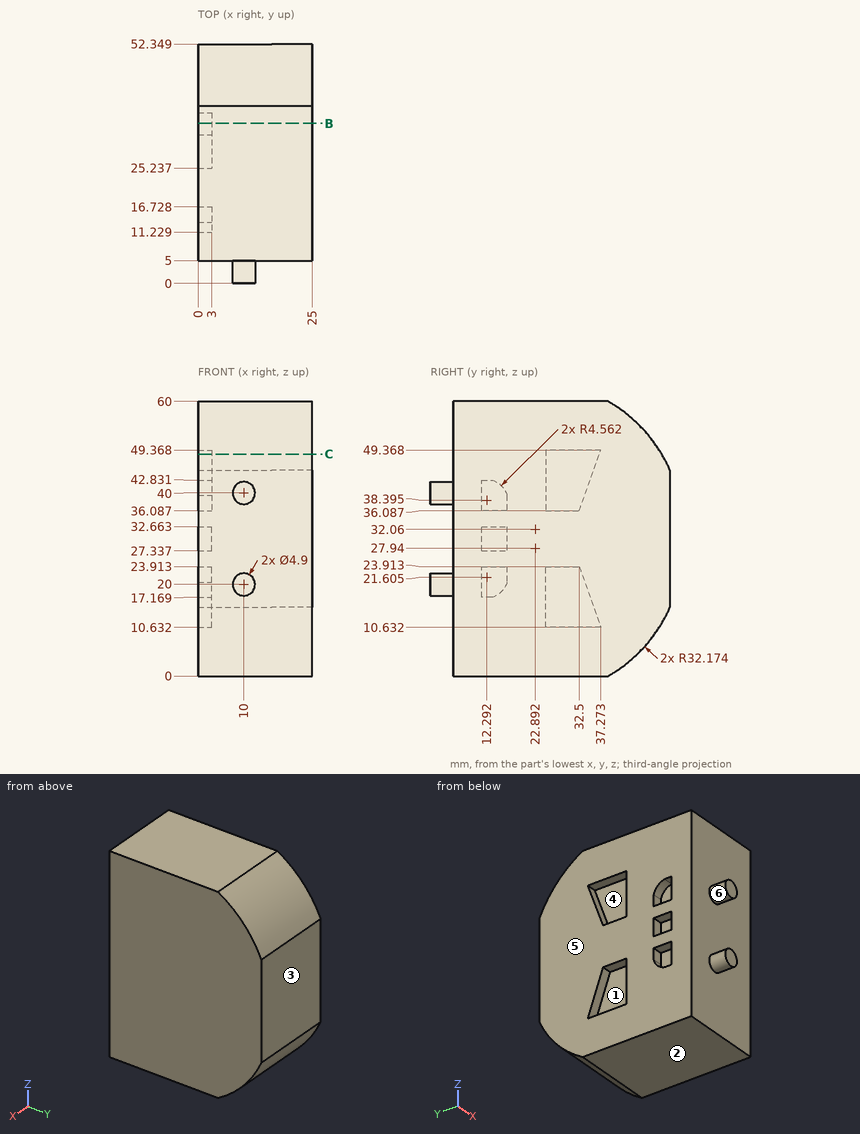
Study the drawing (mm; zero at the part's minimum x, y, z) and answer. A direction names the side the tool comes from. Give positions to 0.01 mm unless a question says otherwise; leave off trailing zeros. Loops run counter-clockwise (first coordinate to the right, second up) from the corner with the lowest first, then second, coordinate; pieces in that order, holes last. Notation, with made-up numbers: (-21, 84.25) - (-8, 84.25) arc R15 ccw to (-8, 109.25) - close; hole circle Ø4 at (55, 18). An arc over 180 degrees is marked (long way). Return JSON: item names as keys, results as strings. Group by question number.
1. Given pin 1 Ø1.5 at (x, z) = (13.5, 30.5) entering from -Y; pin 2 Ø3.5 at (y, z) = (31.5, 41) entering from -X; pin 3 Ø2 at (x, z) = (14, 46.5) entering from +Y (1 decimal), each flat-ended and moving along its own axis, determine where each tip first touches the part or whether it passes through.
2. Straight lines are drawn through the part: line 1 (Y direction, x = 2.25, z = 37.5); line 2 (Y direction, x = 2, z = 11) (1 decimal); line 3 (Y direction, x = 21.5, z = 31.5). For each, find the intervals that lie inside material, in ascending order. Write a range as [from, to].
3. Which of the six approach directions +Z, -Z, +X, -X, +Y, -Y give full straight-line access (tool end or side, diameter ignored) to the marked faces 4, 5 and 6?
4. Find section B-B (y = 35). Write down the section's boundary in (x, z), then the cut area to 3 significant figures.
5. Determine the mould class of the marked faces 1, 2 and 3 for opening direction Y: pulls with the +Y half, pulls with the -Y half, needs draft (parallel to the pull), parting line crosses it, or undercut.
6. Find section C-C (z = 48.5). Write down the section's boundary in (x, y), then the cut area to 3 significant figures.
Verdict:
{
 "1": {"pin 1": "stops at y = 5", "pin 2": "stops at x = 3", "pin 3": "stops at y = 52.1"},
 "2": {"line 1": "y = [5, 11.23], [16.73, 25.24], [33.01, 52.35]", "line 2": "y = [5, 25.2], [37.1, 50.2]", "line 3": "y = [5, 52.35]"},
 "3": {"face 4": "-X", "face 5": "+Z, -Z, -X, +Y, -Y", "face 6": "-Y"},
 "4": {"outline": "(0, 0) - (25, 0) - (25, 60) - (0, 60) - (0, 49.37) - (3, 49.37) - (3, 43.04) - (0, 43.04) - (0, 16.96) - (3, 16.96) - (3, 10.63) - (0, 10.63) - close", "area": "1,460 mm^2"},
 "5": {"face 1": "undercut", "face 2": "needs draft", "face 3": "pulls with the +Y half"},
 "6": {"outline": "(0, 5) - (25, 5) - (25, 50.55) - (0, 50.55) - (0, 36.96) - (3, 36.96) - (3, 25.24) - (0, 25.24) - close", "area": "1,100 mm^2"}
}
